Input: part model. Units: mm. Frame: model coordinates. A direction names the side the tool comes from. Round coordinates to 2 decimals unless told otherwise and drop trailing zeros. Loops run counter-clockwise (first coordinate to the right, second up) from the corner with the lowest first, then second, coordinate; pieces in that order, holes last. Notation, with made-up numbers: (89.5, 4) -> (140.5, 4) arc R15 ccw to (140.5, 13) -> close; hole circle Ø4 at (52.25, -3). An arc over 180 degrees is marked (long way). Answer as a JSON object with one key per item and string values.
```python
from build123d import *

# Parameters (mm, degrees)
F0_R     = 37
F0_R_2   = 2.65
F0_R_3   = 4
F1_DEPTH = 6
F2_DEPTH = 4
F3_DEPTH = 2
F4_SIZE2 = 2.3
F4_SIZE  = 5
F5_R     = 1.3130068335
F6_DEPTH = 1


with BuildPart() as f1:
    # F0 (on Right) → F1 (new body)
    with BuildSketch(Plane.YZ):
        Circle(F0_R)
        with BuildLine():
            Line((-23.0952370323, 14.180454946), (-17.0328632471, 23.8484731203))
            ThreePointArc((-17.0328632471, 23.8484731203), (0.0002590164, 33.2703478915), (17.0295377344, 23.8415279974))
            Line((17.0295377344, 23.8415279974), (23.0899184639, 14.167925942))
            ThreePointArc((23.0899184639, 14.167925942), (23.4636524397, 13.5467460522), (23.8147430167, 12.9124929901))
            Line((23.8147430167, 12.9124929901), (29.162137778, 2.827248294))
            ThreePointArc((29.162137778, 2.827248294), (28.813095975, -16.6349496309), (12.1369519401, -26.6751288313))
            Line((12.1369519401, -26.6751288313), (0.7330157043, -27.0912894495))
            ThreePointArc((0.7330157043, -27.0912894495), (0, -27.1046598669), (-0.7330157043, -27.0912894495))
            Line((-0.7330157043, -27.0912894495), (-12.1441739659, -26.6748652799))
            ThreePointArc((-12.1441739659, -26.6748652799), (-28.8182692269, -16.6382354957), (-29.1731979579, 2.8202694775))
            Line((-29.1731979579, 2.8202694775), (-23.8282527367, 12.9108345034))
            ThreePointArc((-23.8282527367, 12.9108345034), (-23.4733240056, 13.5523299334), (-23.0952370323, 14.180454946))
        make_face(mode=Mode.SUBTRACT)
        with BuildLine():
            ThreePointArc((17.0295377344, 23.8415279974), (0.0002590164, 33.2703478915), (-17.0328632471, 23.8484731203))
            Line((-17.0328632471, 23.8484731203), (-23.0952370323, 14.180454946))
            ThreePointArc((-23.0952370323, 14.180454946), (-23.4733240056, 13.5523299334), (-23.8282527367, 12.9108345034))
            Line((-23.8282527367, 12.9108345034), (-29.1731979579, 2.8202694775))
            ThreePointArc((-29.1731979579, 2.8202694775), (-28.8182692269, -16.6382354957), (-12.1441739659, -26.6748652799))
            Line((-12.1441739659, -26.6748652799), (-0.7330157043, -27.0912894495))
            ThreePointArc((-0.7330157043, -27.0912894495), (0, -27.1046598669), (0.7330157043, -27.0912894495))
            Line((0.7330157043, -27.0912894495), (12.1369519401, -26.6751288313))
            ThreePointArc((12.1369519401, -26.6751288313), (28.813095975, -16.6349496309), (29.162137778, 2.827248294))
            Line((29.162137778, 2.827248294), (23.8147430167, 12.9124929901))
            ThreePointArc((23.8147430167, 12.9124929901), (23.4636524397, 13.5467460522), (23.0899184639, 14.167925942))
            Line((23.0899184639, 14.167925942), (17.0295377344, 23.8415279974))
        make_face()
        with BuildLine():
            Line((-14.5383641102, 8.8148297318), (-8.4759903249, 18.482847906))
            ThreePointArc((-8.4759903249, 18.482847906), (-0.0018003141, 23.1703476982), (8.4704774851, 18.4793926211))
            Line((8.4704774851, 18.4793926211), (14.5308582146, 8.8057905657))
            ThreePointArc((14.5308582146, 8.8057905657), (14.7167955123, 8.4967458506), (14.8914674376, 8.1811970698))
            Line((14.8914674376, 8.1811970698), (20.2388621989, -1.9040476263))
            ThreePointArc((20.2388621989, -1.9040476263), (20.0652095641, -11.5867329668), (11.7686206585, -16.5818468966))
            Line((11.7686206585, -16.5818468966), (0.3646844227, -16.9980075148))
            ThreePointArc((0.3646844227, -16.9980075148), (0, -17.0046594636), (-0.3646844227, -16.9980075148))
            Line((-0.3646844227, -16.9980075148), (-11.7758426843, -16.5815833453))
            ThreePointArc((-11.7758426843, -16.5815833453), (-20.0714122995, -11.5882352941), (-20.2479937541, -1.9073872429))
            Line((-20.2479937541, -1.9073872429), (-14.9030485329, 8.183177783))
            ThreePointArc((-14.9030485329, 8.183177783), (-14.7264670782, 8.5023297318), (-14.5383641102, 8.8148297318))
        make_face(mode=Mode.SUBTRACT)
        with BuildLine():
            ThreePointArc((8.4704774851, 18.4793926211), (-0.0018003141, 23.1703476982), (-8.4759903249, 18.482847906))
            Line((-8.4759903249, 18.482847906), (-14.5383641102, 8.8148297318))
            ThreePointArc((-14.5383641102, 8.8148297318), (-14.7264670782, 8.5023297318), (-14.9030485329, 8.183177783))
            Line((-14.9030485329, 8.183177783), (-20.2479937541, -1.9073872429))
            ThreePointArc((-20.2479937541, -1.9073872429), (-20.0714122995, -11.5882352941), (-11.7758426843, -16.5815833453))
            Line((-11.7758426843, -16.5815833453), (-0.3646844227, -16.9980075148))
            ThreePointArc((-0.3646844227, -16.9980075148), (0, -17.0046594636), (0.3646844227, -16.9980075148))
            Line((0.3646844227, -16.9980075148), (11.7686206585, -16.5818468966))
            ThreePointArc((11.7686206585, -16.5818468966), (20.0652095641, -11.5867329668), (20.2388621989, -1.9040476263))
            Line((20.2388621989, -1.9040476263), (14.8914674376, 8.1811970698))
            ThreePointArc((14.8914674376, 8.1811970698), (14.7167955123, 8.4967458506), (14.5308582146, 8.8057905657))
            Line((14.5308582146, 8.8057905657), (8.4704774851, 18.4793926211))
        make_face()
        with Locations((-12.5573683549, -7.25)):
            Circle(F0_R_2, mode=Mode.SUBTRACT)
        with Locations((12.5573683549, -7.25)):
            Circle(F0_R_2, mode=Mode.SUBTRACT)
        Circle(F0_R_3, mode=Mode.SUBTRACT)
        with Locations((0, 14.5)):
            Circle(F0_R_2, mode=Mode.SUBTRACT)
    extrude(amount=-F1_DEPTH)

    # F0 (on Right) → F2 (cut)
    with BuildSketch(Plane.YZ):
        with BuildLine():
            ThreePointArc((17.0295377344, 23.8415279974), (0.0002590164, 33.2703478915), (-17.0328632471, 23.8484731203))
            Line((-17.0328632471, 23.8484731203), (-23.0952370323, 14.180454946))
            ThreePointArc((-23.0952370323, 14.180454946), (-23.4733240056, 13.5523299334), (-23.8282527367, 12.9108345034))
            Line((-23.8282527367, 12.9108345034), (-29.1731979579, 2.8202694775))
            ThreePointArc((-29.1731979579, 2.8202694775), (-28.8182692269, -16.6382354957), (-12.1441739659, -26.6748652799))
            Line((-12.1441739659, -26.6748652799), (-0.7330157043, -27.0912894495))
            ThreePointArc((-0.7330157043, -27.0912894495), (0, -27.1046598669), (0.7330157043, -27.0912894495))
            Line((0.7330157043, -27.0912894495), (12.1369519401, -26.6751288313))
            ThreePointArc((12.1369519401, -26.6751288313), (28.813095975, -16.6349496309), (29.162137778, 2.827248294))
            Line((29.162137778, 2.827248294), (23.8147430167, 12.9124929901))
            ThreePointArc((23.8147430167, 12.9124929901), (23.4636524397, 13.5467460522), (23.0899184639, 14.167925942))
            Line((23.0899184639, 14.167925942), (17.0295377344, 23.8415279974))
        make_face()
        with BuildLine():
            Line((-14.5383641102, 8.8148297318), (-8.4759903249, 18.482847906))
            ThreePointArc((-8.4759903249, 18.482847906), (-0.0018003141, 23.1703476982), (8.4704774851, 18.4793926211))
            Line((8.4704774851, 18.4793926211), (14.5308582146, 8.8057905657))
            ThreePointArc((14.5308582146, 8.8057905657), (14.7167955123, 8.4967458506), (14.8914674376, 8.1811970698))
            Line((14.8914674376, 8.1811970698), (20.2388621989, -1.9040476263))
            ThreePointArc((20.2388621989, -1.9040476263), (20.0652095641, -11.5867329668), (11.7686206585, -16.5818468966))
            Line((11.7686206585, -16.5818468966), (0.3646844227, -16.9980075148))
            ThreePointArc((0.3646844227, -16.9980075148), (0, -17.0046594636), (-0.3646844227, -16.9980075148))
            Line((-0.3646844227, -16.9980075148), (-11.7758426843, -16.5815833453))
            ThreePointArc((-11.7758426843, -16.5815833453), (-20.0714122995, -11.5882352941), (-20.2479937541, -1.9073872429))
            Line((-20.2479937541, -1.9073872429), (-14.9030485329, 8.183177783))
            ThreePointArc((-14.9030485329, 8.183177783), (-14.7264670782, 8.5023297318), (-14.5383641102, 8.8148297318))
        make_face(mode=Mode.SUBTRACT)
    extrude(amount=-F2_DEPTH, mode=Mode.SUBTRACT)

    # F3 (add): a face of the model
    f3_faces = [f1.faces().sort_by_distance(p)[0] for p in [
        (0, -6.0488520011, -16.2030604824),
    ]]
    extrude(f3_faces, amount=F3_DEPTH)

    # F4
    f4_edges = [f1.edges().sort_by_distance(p)[0] for p in [
        (-6, -2.65, 14.5),
        (-6, 9.907368, -7.25),
        (-6, -15.207368, -7.25),
    ]]
    f4_side = f1.faces().sort_by_distance((-6, -35.953482, 0))[0]
    chamfer(f4_edges, length=F4_SIZE, length2=F4_SIZE2, reference=f4_side)

    # F5 (on face) → F6 (cut)
    with BuildSketch(Plane(origin=(-6, 0, 0), x_dir=(0, -1, 0), z_dir=(-1, 0, 0))):
        with Locations((0, 25.6734099239)):
            Circle(F5_R)
    extrude(amount=-F6_DEPTH, mode=Mode.SUBTRACT)


solid = f1.part
```
1) Section C-C, the plane z = 32. Output: boundary loops of the cut face in (x, y), plus the area to 3 significant figures.
Output:
{"outline": "(-6, -18.57) -> (0, -18.57) -> (0, -7.04) -> (-4, -7.04) -> (-4, 7.03) -> (0, 7.03) -> (0, 18.57) -> (-6, 18.57) -> close", "area": "167 mm^2"}
2) Section B-B, the plane z = -7.25. Output: boundary loops of the cut face in (x, y), plus the area to 3 significant figures.
Output:
{"outline": "(-6, -36.28) -> (0, -36.28) -> (0, -31.5) -> (-4, -31.5) -> (-4, -21.39) -> (2, -21.39) -> (2, -15.21) -> (-3.7, -15.21) -> (-6, -20.21) -> close; (-6, -4.91) -> (-3.7, -9.91) -> (2, -9.91) -> (2, 9.91) -> (-3.7, 9.91) -> (-6, 4.91) -> close; (-6, 20.21) -> (-3.7, 15.21) -> (2, 15.21) -> (2, 21.38) -> (-4, 21.38) -> (-4, 31.49) -> (0, 31.49) -> (0, 36.28) -> (-6, 36.28) -> close", "area": "332 mm^2"}
3) Section A-A, the plane x = -2. Count the separate pieces of the cut face and the enclosed holes in it, plus the area to 3 significant figures.
Output:
{"separate pieces": "2", "enclosed holes": "5", "area": "2,540 mm^2"}
4) Ray query, probe 1 along Z at (x, y) = (-0.9, 0); probe 2 along Z at (x, y) = (-2, 14); probe 3 along Y at (x, z) = (-3.5, 10). Return the intervals inside material, ascending.
Output:
{"probe 1": "z = -37 to -27.1, -17 to -4, 4 to 11.85, 17.15 to 23.17, 33.27 to 37", "probe 2": "z = -34.25 to -26.52, -16.25 to -9.47, -5.03 to 9.65, 27.59 to 34.25", "probe 3": "y = -35.62 to -25.37, -13.8 to 13.78, 25.36 to 35.62"}
5) Contact query for flat-ended pins moving along their axis: P1, Ø7, axis at y = -12.56, z = -7.25, coming from the -X side; P2, Ø5, axis at y = 0, z = 14.5, coming from the +X side; P3, Ø1.5, axis at x = -1.5, y = 8, coming from the +Z side; P4, Ø1, axis at x = 0, y = -27.5, coming from the -Z side. Output: stop coordinate, or through.
Output:
{"P1": "stops at x = -4.09", "P2": "passes through", "P3": "stops at z = 36.28", "P4": "stops at z = -25.3"}
6) Reachability of faces 3 (the face through (-5.51, 0.28, 24.39)), 4 (the face through (-6, -1, -8)), 5 (the face through (-1.04, -20, -11.71)) from +Z, -Z, +X, -X, +Y, -Y: full face, straight path, thin tool, end or side. Return the list, or none.
Output:
{"face 3": "-X", "face 4": "+Z, -Z, -X, +Y, -Y", "face 5": "+X"}
7) Section D-D, the plane z = -30. Output: boundary loops of the cut face in (x, y), plus the area to 3 significant figures.
Output:
{"outline": "(-6, -21.66) -> (0, -21.66) -> (0, 21.66) -> (-6, 21.66) -> close", "area": "260 mm^2"}
8) Draft query along Z for faces 1 (the face through (-1.97, 0.28, 33.27)), 2 (the face through (0, -22, 17)). Return one class per face: +Z half, -Z half, draft (parallel to the pull), parting line (faces both ways), or undercut.
Output:
{"face 1": "undercut", "face 2": "draft"}
